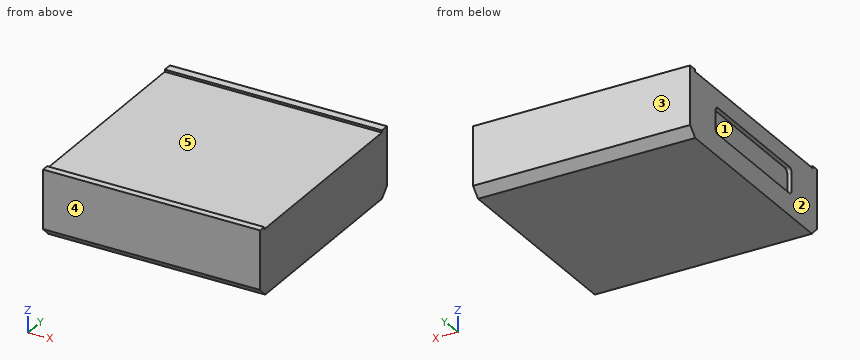
```python
from build123d import *

# Parameters (mm, degrees)
F0_W     = 50
F0_H     = 50
F1_DEPTH = 15
F2_SIZE  = 2
F3_W     = 30
F3_H     = 5.985749
F4_DEPTH = 1
F5_R     = 1
F6_W     = 50
F6_H     = 2
F6_H_2   = 1.608082
F7_DEPTH = 0.5


with BuildPart() as f1:
    # F0 (on Top) → F1 (new body)
    with BuildSketch(Plane.XY):
        with Locations((25, 25)):
            Rectangle(F0_W, F0_H)
    extrude(amount=F1_DEPTH)

    # F2
    f2_edges = [f1.edges().sort_by_distance(p)[0] for p in [
        (25, 0, 0),
        (25, 50, 0),
    ]]
    chamfer(f2_edges, length=F2_SIZE)

    # F3 (on face) → F4 (cut)
    with BuildSketch(Plane(origin=(0, 0, 0), x_dir=(0, -1, 0), z_dir=(-1, 0, 0))):
        with Locations((-25, 8.007126)):
            Rectangle(F3_W, F3_H)
    extrude(amount=-F4_DEPTH, mode=Mode.SUBTRACT)

    # F5
    f5_edges = [f1.edges().sort_by_distance(p)[0] for p in [
        (0.5, 40, 11),
        (0.5, 40, 5.014251),
        (0.5, 10, 11),
        (0.5, 10, 5.014251),
    ]]
    fillet(f5_edges, radius=F5_R)

    # F6 (on face) → F7 (join)
    with BuildSketch(Plane.XY.offset(15)):
        with Locations((25, 49)):
            Rectangle(F6_W, F6_H)
        with Locations((25, 0.804041)):
            Rectangle(F6_W, F6_H_2)
    extrude(amount=F7_DEPTH)


solid = f1.part
```
The listing builds one solid part. Answer for the finished solid, in the listing's coordinates (mm). Face numbers are marked on the shaded views. A direction names the side the tool comes from. Give positions to 0.01 mm unless a question says otherwise; leave off trailing zeros. Order: outer loops, then holes, each group sorted by start corner. A loop starts at its lowest first (then second) coordinate and runs counter-clockwise, first axis right, second up.
1) Find section B-B on y = 12. Write down the section's boundary in (x, z), then the cut area to 3 significant figures.
Reported:
outline: (0, 0) - (50, 0) - (50, 15) - (0, 15) - (0, 11) - (1, 11) - (1, 5.01) - (0, 5.01) - close
area: 744 mm2
2) Consider line 1 along Z through (x, y) = (11, 32.5); line 2 along X through (y, z) = (36, 8.25). Determine where each line is inside the solid, lowest interval first.
Reported:
line 1: z = 0 to 15
line 2: x = 1 to 50
3) Determine the mould class of the marked faces 1, 2 and 3 for opening direction Y: pulls with the +Y half, pulls with the -Y half, needs draft (parallel to the pull), parting line crosses it, or undercut.
Reported:
face 1: undercut
face 2: needs draft
face 3: pulls with the +Y half
4) For the marked faces 4 and 5, determine the directions among +Z, -Z, +X, -X, +Y, -Y from which every point of the face is accessible in a straight line to the end or side of a thin tool.
Reported:
face 4: +Z, -Z, +X, -X, -Y
face 5: +Z, +X, -X
5) Find section A-A on x = 13. Write down the section's boundary in (y, z), then the cut area to 3 significant figures.
Reported:
outline: (0, 2) - (2, 0) - (48, 0) - (50, 2) - (50, 15.5) - (48, 15.5) - (48, 15) - (1.61, 15) - (1.61, 15.5) - (0, 15.5) - close
area: 748 mm2
6) Given P1, Ø2, axis at x = 45, y = 10.5, coming from the +Z side; P2, Ø1.5, axis at y = 23.5, z = 7, coming from the -X side, each flat-ended and moving along its own axis, determine where each tip first touches the part or whether it passes through.
Reported:
P1: stops at z = 15
P2: stops at x = 1
7) Find section C-C on y = 4. Write down the section's boundary in (x, z).
Reported:
outline: (0, 0) - (50, 0) - (50, 15) - (0, 15) - close
